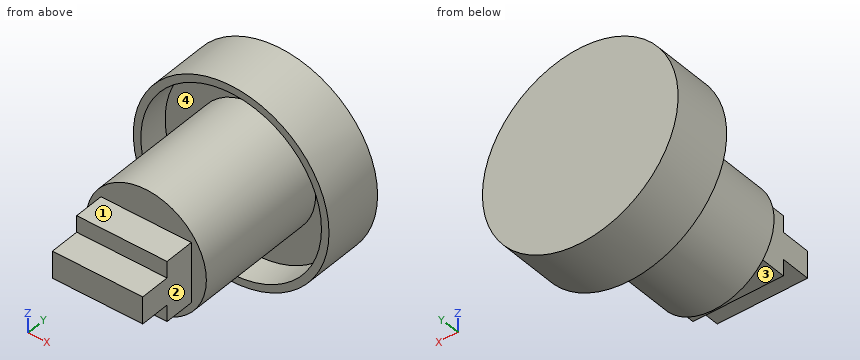
```python
from build123d import *

# Parameters (mm, degrees)
F0_R     = 41.275
F1_DEPTH = 25.4
F2_R     = 38.1
F3_DEPTH = 12.7
F4_R     = 25.4
F5_DEPTH = 57.15
F6_W     = 38.1
F6_H     = 25.4
F7_DEPTH = 25.4
F8_W     = 38.1
F8_H     = 6.987833
F8_H_2   = 6.985
F9_DEPTH = 12.7


with BuildPart() as f1:
    # F0 (on Front) → F1 (new body)
    with BuildSketch(Plane.XZ):
        Circle(F0_R)
    extrude(amount=F1_DEPTH)

    # F2 (on face) → F3 (cut)
    with BuildSketch(Plane.XZ.offset(25.4)):
        Circle(F2_R)
    extrude(amount=-F3_DEPTH, mode=Mode.SUBTRACT)

    # F4 (on face) → F5 (join)
    with BuildSketch(Plane.XZ.offset(12.7)):
        Circle(F4_R)
    extrude(amount=F5_DEPTH)

    # F6 (on face) → F7 (join)
    with BuildSketch(Plane.XZ.offset(69.85)):
        Rectangle(F6_W, F6_H)
    extrude(amount=F7_DEPTH)

    # F8 (on face) → F9 (cut)
    with BuildSketch(Plane.XZ.offset(95.25)):
        with Locations((0, 9.206084)):
            Rectangle(F8_W, F8_H)
        with Locations((0, -9.2075)):
            Rectangle(F8_W, F8_H_2)
    extrude(amount=-F9_DEPTH, mode=Mode.SUBTRACT)


solid = f1.part
```
Here's how the part is built. I have some questions about the finished solid (model axes, mm). Face numbers are marked on the shaded views. A direction names the side the tool comes from. Coordinates: 2 decimals unless noted, no trailing zeros. Order: outer loops, then holes, each group sorted by start corner. A loop starts at its lowest first (then second) coordinate and runs counter-clockwise, first axis right, second up.
1) Imagine slicing it at C-C on z = 0. List the corners of the cut face in (x, y) for me (3 decimals), and give its area (3 significant figures).
2) Imagine slicing it at B-B on x = 0. List the corners of the cut face in (y, z) for me (3 decimals), and give its area (3 significant figures).
3) Will these pins go through, and if not, where does the flat tip stop? pin 1 (4 mm diameter, centred on x = 2.5, y = -74.5, fed in from -Z); pin 2 (10 mm diameter, centred on x = 7.5, y = -92, fed in from -Z) (3 decimals); pin 3 (12.5 mm diameter, centred on y = -83.5, z = -0.5, fed in from -X).
4) Imagine slicing it at D-D on y = -10.5. List the corners of the cut face in (x, z) for me (3 decimals).
5) I need wall thicknesses on line 1 (Z direction, x = 0, y = -15.5) (3 decimals); line 2 (X direction, y = -19.5, z = -1); line 3 (Y direction, x = -36, z = 1.5). Which ranges of each line are inside material? Lowest first, please.
6) Which directions (+Z, -Z, +X, -X, +Y, -Y) give clear straight access to the entire face, cutting with the end or side of a thin tool? Please do the marked faces 1, 2, 3 and 4.
7) Imagine slicing it at A-A on y = -20.5. List the corners of the cut face in (x, z) for me (3 decimals), and give its area (3 significant figures).
Response values:
1. outline: (-41.275, -25.4) - (-38.1, -25.4) - (-38.1, -12.7) - (-25.4, -12.7) - (-25.4, -69.85) - (-19.05, -69.85) - (-19.05, -95.25) - (19.05, -95.25) - (19.05, -69.85) - (25.4, -69.85) - (25.4, -12.7) - (38.1, -12.7) - (38.1, -25.4) - (41.275, -25.4) - (41.275, 0) - (-41.275, 0) - close
1. area: 5,000 mm2
2. outline: (-95.25, -5.715) - (-82.55, -5.715) - (-82.55, -12.7) - (-69.85, -12.7) - (-69.85, -25.4) - (-12.7, -25.4) - (-12.7, -38.1) - (-25.4, -38.1) - (-25.4, -41.275) - (0, -41.275) - (0, 41.275) - (-25.4, 41.275) - (-25.4, 38.1) - (-12.7, 38.1) - (-12.7, 25.4) - (-69.85, 25.4) - (-69.85, 12.7) - (-82.55, 12.7) - (-82.55, 5.712) - (-95.25, 5.712) - close
2. area: 4,500 mm2
3. pin 1: stops at z = -12.7
3. pin 2: stops at z = -5.715
3. pin 3: stops at x = -19.05
4. outline: circle Ø82.55 at (0, 0)
5. line 1: z = -41.275 to -38.1, -25.4 to 25.4, 38.1 to 41.275
5. line 2: x = -41.26 to -38.09, -25.38 to 25.38, 38.09 to 41.26
5. line 3: y = -12.7 to 0
6. face 1: +Z, +X, -X, -Y
6. face 2: +Z, -Z, +X, -Y
6. face 3: -Z, +X, -X, -Y
6. face 4: -Y
7. outline: circle Ø82.55 at (0, 0); circle Ø50.8 at (0, 0); hole circle Ø76.2 at (0, 0)
7. area: 2,820 mm2
